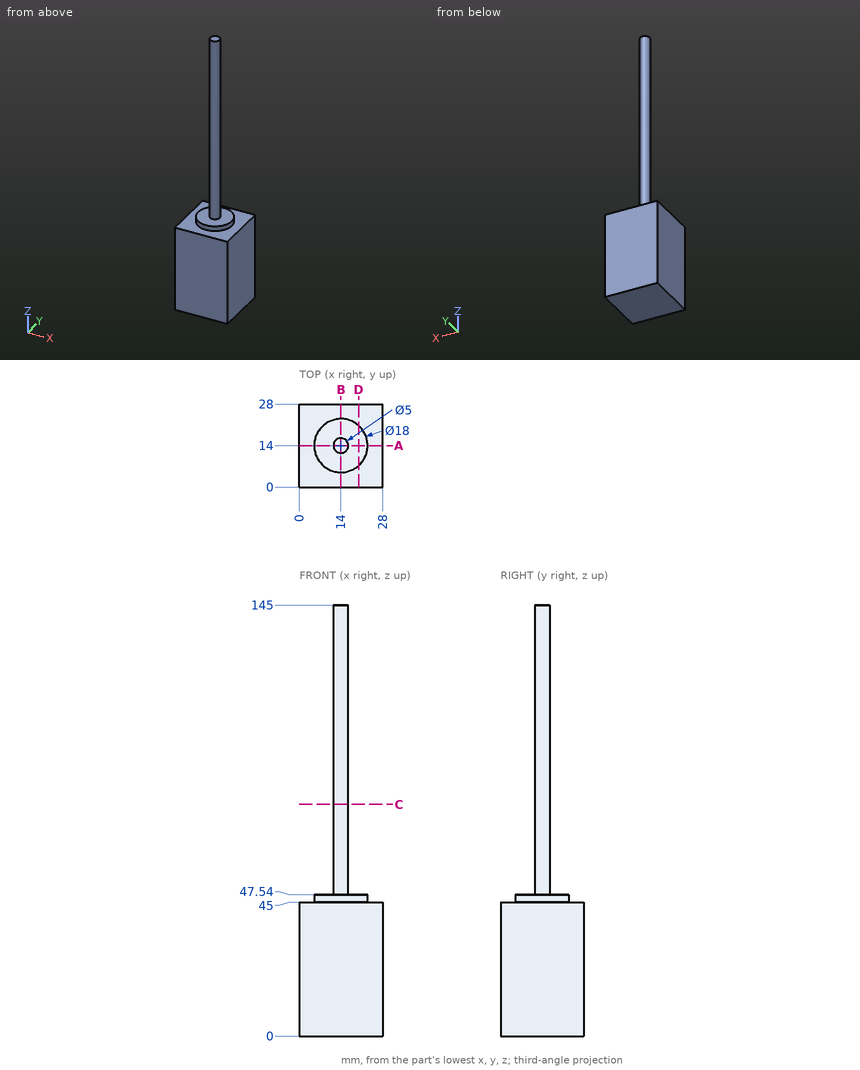
Answer from the drawing. Dimensions are ordinates in mm from the lowest x, y and z of the part. Give positions to 0.01 mm unless a question says otherwise; leave off trailing zeros. Loops run counter-clockwise (first coordinate to the right, second up) from the corner with the lowest first, then second, coordinate; pieces in that order, holes last. Notation, with made-up numbers: (18.5, 60) - (70.5, 60) arc R19 ccw to (70.5, 92) - close; hole circle Ø10 at (-35.5, 2.25). An arc over 180 degrees is marked (long way). Answer as a JSON object with one key per item and string values.
1. Flat-ended cylindrical pins translate along their axes: pin 1 Ø10 at (y, z) = (8, 70.5) entering from -X; pin 2 Ø8 at (x, y) = (21, 14.5) entering from +Z; pin 3 Ø1 at (x, y) = (24, 24.5) entering from +Z. Find the tip coordinate at first contact, or state that the pin passes through.
Determined:
{"pin 1": "x = 11.71", "pin 2": "z = 47.54", "pin 3": "z = 45"}
2. A cutting plane is placed at D-D (x = 20). Write down the section's boundary in (y, z), then the cut area to 3 significant figures.
Determined:
{"outline": "(0, 0) - (28, 0) - (28, 45) - (20.71, 45) - (20.71, 47.54) - (7.29, 47.54) - (7.29, 45) - (0, 45) - close", "area": "1,290 mm²"}
3. Find the intervals of material crossed by L1, parallel to Z at x = 8, y = 16.5; L2, parallel to Z at x = 9.25, y = 4.5; L3, parallel to Y at x = 11.75, z = 119.5, in increasing order. Write a range as [from, to].
Determined:
{"L1": "[0, 47.54]", "L2": "[0, 45]", "L3": "[12.91, 15.09]"}
4. A cutting plane is placed at C-C (z = 78). Write down the section's boundary in (x, y).
Determined:
{"outline": "circle Ø5 at (14, 14)"}
5. A cutting plane is placed at A-A (y = 14). Write down the section's boundary in (x, z).
Determined:
{"outline": "(0, 0) - (28, 0) - (28, 45) - (23, 45) - (23, 47.54) - (16.5, 47.54) - (16.5, 145) - (11.5, 145) - (11.5, 47.54) - (5, 47.54) - (5, 45) - (0, 45) - close"}
